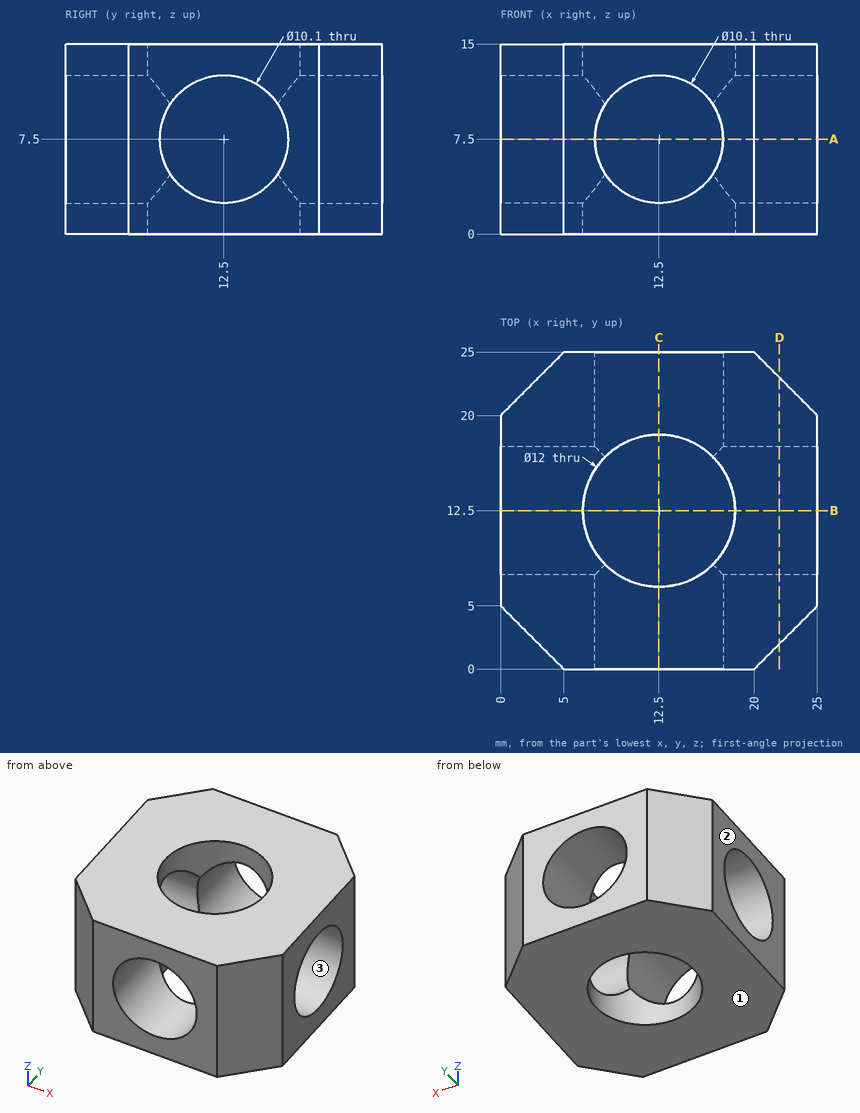
Could you check a few things on this drawing? It's one solid part, dimensions in mm from its lowest x, y, z. Give positions to 0.01 mm unless a question says otherwise; leave off trailing zeros. Write each loop counter-clockwise with the first axis right and the second up, starting at its lowest first coordinate (ties: lowest second). Pieces come first, ordered by that corner, then holes.
(1) Imagine slicing it at D-D, the plane x = 22. Write out the boundary of the cut face in (y, z).
Output values:
outline: (2, 0) - (23, 0) - (23, 15) - (2, 15) - close; hole circle Ø10.1 at (12.5, 7.5)
(2) Imagine slicing it at B-B, the plane y = 12.5. Write out the boundary of the cut face in (x, z), and give its area (3 significant figures).
Output values:
outline: (0, 0) - (6.5, 0) - (6.5, 2.45) - (0, 2.45) - close; (0, 12.55) - (6.5, 12.55) - (6.5, 15) - (0, 15) - close; (18.5, 0) - (25, 0) - (25, 2.45) - (18.5, 2.45) - close; (18.5, 12.55) - (25, 12.55) - (25, 15) - (18.5, 15) - close
area: 63.7 mm2
(3) If I drill on L1, parallel to Z at x = 12.5, y = 5; L2, parallel to Y at x = 18.5, z = 7.5; L3, parallel to Y at x = 16.5, z = 4.25, over which ranges is the centre line in solid material (lowest first)?
Output values:
L1: z = 0 to 2.45, 12.55 to 15
L2: y = 0 to 7.45, 17.55 to 25
L3: y = 0 to 8.03, 16.97 to 25
(4) Will this pin go through, and if not, where does the flat tip stop? pin 1 (12 mm diameter, centred on x = 11.5, y = 17, fed in from -Z).
Output values:
pin 1: stops at z = 0
(5) Imagine slicing it at A-A, the plane z = 7.5. Write out the boundary of the cut face in (x, y).
Output values:
outline: (0, 5) - (5, 0) - (7.45, 0) - (7.45, 7.45) - (0, 7.45) - close; (0, 17.55) - (7.45, 17.55) - (7.45, 25) - (5, 25) - (0, 20) - close; (17.55, 0) - (20, 0) - (25, 5) - (25, 7.45) - (17.55, 7.45) - close; (17.55, 17.55) - (25, 17.55) - (25, 20) - (20, 25) - (17.55, 25) - close
(6) Thinking about a two-plate mould opening in Z: for the marked faces 1, 2 and 3, which applies, pulls with the +Z half, pulls with the -Z half, needs draft (parallel to the pull), parting line crosses it, or undercut?
Output values:
face 1: pulls with the -Z half
face 2: needs draft
face 3: undercut
